For this review, take the finished solid that the model builds, in its own axes (mm). A direction names the side the tool comes from. Give positions to 0.01 mm unless a question says otherwise; leave off trailing zeros. Loops run counter-clockwise (first coordinate to the right, second up) from the corner with the lowest first, then second, coordinate; pieces in that order, holes last. Notation, with made-up numbers: (71, 32.5) -> (94, 32.5) arc R22 ccw to (94, 56.5) -> close; hole circle Ø10 at (74, 89.25). An arc over 180 degrees is marked (long way). One line per question, with ' | ' between items. Start each with the question number.
(1) Tool access review of faces 4 (the flat face through (20, 0, 1)), 5 (the flat face through (-1.12, -23.72, 1.48)): name each direction out of +Z, -Z, +X, -X, +Y, -Y from which nothing blocks a thin tool from reaching the whole face with its end or side.
(2) Consider section D-D (x = 15). Write out the cut boundary in (y, z).
(3) Consider section C-C (z = 0.7). Write out the cut boundary in (x, y).
(4) Consider section B-B (x = 24). Write out the cut boundary in (y, z), and give its area (3 significant figures).
(5) Draft analysis for pull direction X (two halves, no side actions). For faces 1 (the flat face through (40, -10, 1)), 2 (the cylindrical face through (-9.441, -20.414, 1.521)), 3 (the cylindrical face through (49.1, 5.14, 1.52)), state which applies: +X half, -X half, draft (parallel to the pull), parting line (faces both ways), or undercut.
(6) Wall thickness on probe 1 along Y at (x, z) = (44.7, 2); probe 2 along Y at (x, z) = (35, 2.3); probe 3 along Y at (x, z) = (12, 1.9): over which ranges is each line inside the solid? List them lowest first.
(7) Consider section A-A (y = -15). Write out the cut boundary in (x, z), and give its area (3 significant figures).
from build123d import *

# Parameters (mm, degrees)
SKETCH_1_W          = 60
SKETCH_1_H          = 32
SKETCH_1_R          = 1.5
SKETCH_1_W_2        = 40
SKETCH_1_H_2        = 20
EXTRUDE_1_DEPTH     = 3
SKETCH_2_R          = 1.5
CUT_EXTRUDE_1_DEPTH = 3
FILLET_1_R          = 3
CUT_EXTRUDE_2_DEPTH = 10
FILLET_2_R          = 3


with BuildPart() as part:
    # 草图1 → 凸台-拉伸1 (new body)
    with BuildSketch(Plane.XY):
        with Locations((20, -10)):
            Rectangle(SKETCH_1_W, SKETCH_1_H)
        with Locations((-4.7, -5)):
            Circle(SKETCH_1_R, mode=Mode.SUBTRACT)
        with Locations((-4.7, -15)):
            Circle(SKETCH_1_R, mode=Mode.SUBTRACT)
        with Locations((44.7, -5)):
            Circle(SKETCH_1_R, mode=Mode.SUBTRACT)
        with Locations((44.7, -15)):
            Circle(SKETCH_1_R, mode=Mode.SUBTRACT)
        with Locations((35, -23)):
            Circle(SKETCH_1_R, mode=Mode.SUBTRACT)
        with Locations((15, -23)):
            Circle(SKETCH_1_R, mode=Mode.SUBTRACT)
        with Locations((20, -10)):
            Rectangle(SKETCH_1_W_2, SKETCH_1_H_2, mode=Mode.SUBTRACT)
    extrude(amount=EXTRUDE_1_DEPTH)

    # 草图2 → 切除-拉伸1 (cut)
    with BuildSketch(Plane.XY.offset(3)):
        with Locations((1.5, 0)):
            Circle(SKETCH_2_R)
        with Locations((38.5, 0)):
            Circle(SKETCH_2_R)
        with Locations((38.5, -20)):
            Circle(SKETCH_2_R)
        with Locations((1.5, -20)):
            Circle(SKETCH_2_R)
    extrude(amount=-CUT_EXTRUDE_1_DEPTH, mode=Mode.SUBTRACT)

    # 圆角1
    fillet_1_edges = [part.edges().sort_by_distance(p)[0] for p in [
        (-10, 6, 1.5),
        (50, 6, 1.5),
        (50, -26, 1.5),
        (-10, -26, 1.5),
    ]]
    fillet(fillet_1_edges, radius=FILLET_1_R)

    # 草图3 → 切除-拉伸2 (cut)
    with BuildSketch(Plane(origin=(0, 0, 0), x_dir=(-1, 0, 0), z_dir=(0, 0, -1))):
        Polygon((-5.9461814, -26), (10, -20.853371157), (15.489211813, -37.273669186), align=None)
    extrude(amount=-CUT_EXTRUDE_2_DEPTH, mode=Mode.SUBTRACT)

    # 圆角2
    fillet_2_edges = [part.edges().sort_by_distance(p)[0] for p in [
        (5.9461814, -26, 1.5),
        (-10, -20.853371157, 1.5),
    ]]
    fillet(fillet_2_edges, radius=FILLET_2_R)


solid = part.part
A:
1) face 4: +Z, -Z | face 5: +Z, -Z, -X, -Y
2) outline: (-26, 0) -> (-24.5, 0) -> (-24.5, 3) -> (-26, 3) -> close; (-21.5, 0) -> (-20, 0) -> (-20, 3) -> (-21.5, 3) -> close; (0, 0) -> (6, 0) -> (6, 3) -> (0, 3) -> close
3) outline: (-10, -18.67) arc R3 ccw to (-7.92, -21.52) -> (5.5, -25.85) arc R3 ccw to (6.42, -26) -> (47, -26) arc R3 ccw to (50, -23) -> (50, 3) arc R3 ccw to (47, 6) -> (-7, 6) arc R3 ccw to (-10, 3) -> close; hole circle Ø3 at (-4.7, -15); hole circle Ø3 at (-4.7, -5); hole (0, -20) arc R1.5 ccw to (3, -20) -> (37, -20) arc R1.5 ccw to (40, -20) -> (40, 0) arc R1.5 ccw to (37, 0) -> (3, 0) arc R1.5 ccw to (0, 0) -> close; hole circle Ø3 at (15, -23); hole circle Ø3 at (35, -23); hole circle Ø3 at (44.7, -15); hole circle Ø3 at (44.7, -5)
4) outline: (-26, 0) -> (-20, 0) -> (-20, 3) -> (-26, 3) -> close; (0, 0) -> (6, 0) -> (6, 3) -> (0, 3) -> close | area: 36.0 mm^2
5) face 1: undercut | face 2: -X half | face 3: +X half
6) probe 1: y = -26 to -16.5, -13.5 to -6.5, -3.5 to 6 | probe 2: y = -26 to -24.5, -21.5 to -20, 0 to 6 | probe 3: y = -26 to -20, 0 to 6
7) outline: (-10, 0) -> (-6.2, 0) -> (-6.2, 3) -> (-10, 3) -> close; (-3.2, 0) -> (0, 0) -> (0, 3) -> (-3.2, 3) -> close; (40, 0) -> (43.2, 0) -> (43.2, 3) -> (40, 3) -> close; (46.2, 0) -> (50, 0) -> (50, 3) -> (46.2, 3) -> close | area: 42.0 mm^2
